Verification items for the finished model (mm, model axes). A direction names the side the tool comes from. Give positions to 0.01 mm unless a question says otherwise; leave off trailing zeros. Loops run counter-clockwise (first coordinate to the right, second up) from the corner with the lowest first, then second, coordinate; pieces in that order, holes last. Notation, with made-up numbers: M -29,54.5 L -24,54.5 A23 ccw -24,90.5 Z; hole C 72.5,13.25 d9. An arc over 180 degrees is marked long. Answer in a Markdown table with one row per item.
```python
from build123d import *

# Parameters (mm, degrees)
BOSS_EXTRUDE1_DEPTH      = 40
BOSS_EXTRUDE1_DEPTH_BACK = 40
CUT_EXTRUDE1_DEPTH       = 30
CUT_EXTRUDE1_DEPTH_BACK  = 48.5
SKETCH3_R                = 1.5
CUT_EXTRUDE2_DEPTH       = 40.921431767
FILLET1_R                = 1
CUT_EXTRUDE3_DEPTH       = 40
FILLET2_R                = 0.5


with BuildPart() as part:
    # Sketch1 → Boss-Extrude1 (new body, two sides)
    with BuildSketch(Plane(origin=(61.148873397, 0, -61.148873397), x_dir=(0.707106781, 0, 0.707106781), z_dir=(-0.707106781, 0, 0.707106781))) as boss_extrude1_sk:
        Polygon((-3.75, -92.901515315), (-3.75, -84.066578824), (-7.75, -81.757177748), (-7.75, -79.151515315), (3.75, -79.151515315), (3.75, -92.901515315), (3.75, -159.151515315), (-3.75, -159.151515315), align=None)
    extrude(amount=BOSS_EXTRUDE1_DEPTH)
    extrude(boss_extrude1_sk.sketch, amount=-BOSS_EXTRUDE1_DEPTH_BACK)

    # Sketch2 → Cut-Extrude1 (cut, two sides)
    with BuildSketch(Plane(origin=(-2.651650429, 0, -2.651650429), x_dir=(-0.707106781, 0, 0.707106781), z_dir=(-0.707106781, 0, -0.707106781))) as cut_extrude1_sk:
        with BuildLine():
            Line((-83.584702548, -79.151515315), (-83.584702548, -93.901515315))
            ThreePointArc((-83.584702548, -93.901515315), (-95.268174411, -132.944313121), (-126.477566081, -159.151515315))
            Line((-126.477566081, -159.151515315), (-126.477566081, -79.151515315))
            Line((-126.477566081, -79.151515315), (-83.584702548, -79.151515315))
        make_face()
        with BuildLine():
            Line((-65.634702548, -93.901515315), (-65.634702548, -79.151515315))
            Line((-65.634702548, -79.151515315), (-46.477566081, -79.151515315))
            Line((-46.477566081, -79.151515315), (-46.477566081, -159.151515315))
            Line((-46.477566081, -159.151515315), (-103.655823441, -159.151515315))
            ThreePointArc((-103.655823441, -159.151515315), (-75.833406523, -131.661176774), (-65.634702548, -93.901515315))
        make_face()
    extrude(amount=CUT_EXTRUDE1_DEPTH, mode=Mode.SUBTRACT)
    extrude(cut_extrude1_sk.sketch, amount=-CUT_EXTRUDE1_DEPTH_BACK, mode=Mode.SUBTRACT)

    # Sketch3 → Cut-Extrude2 (cut, through all)
    with BuildSketch(Plane(origin=(2.651650429, 0, 2.651650429), x_dir=(0.707106781, 0, -0.707106781), z_dir=(0.707106781, 0, 0.707106781))):
        with Locations((74.128214207, -88.901515315)):
            Circle(SKETCH3_R)
    extrude(amount=-CUT_EXTRUDE2_DEPTH, mode=Mode.SUBTRACT)

    # Fillet1
    fillet1_edges = [part.edges().sort_by_distance(p)[0] for p in [
        (73.295735665, -159.151515315, -73.295735665),
        (89.433144644, -159.151515315, -89.433144644),
    ]]
    fillet(fillet1_edges, radius=FILLET1_R)

    # Sketch4 → Cut-Extrude3 (cut)
    with BuildSketch(Plane(origin=(-2.651650429, 0, -2.651650429), x_dir=(-0.707106781, 0, 0.707106781), z_dir=(-0.707106781, 0, -0.707106781))):
        with BuildLine():
            ThreePointArc((-96.334442354, -150.659659636), (-100.301370683, -153.543969496), (-104.455461262, -156.151515315))
            Line((-104.455461262, -156.151515315), (-114.508069897, -156.151515315))
            ThreePointArc((-114.508069897, -156.151515315), (-107.203125114, -150.779152155), (-100.609312238, -144.554512732))
            Line((-100.609312238, -144.554512732), (-96.334442354, -150.659659636))
        make_face()
        with BuildLine():
            ThreePointArc((-85.691714117, -140.433955852), (-89.676742116, -144.76688928), (-94.002421329, -148.759790428))
            Line((-94.002421329, -148.759790428), (-98.550711636, -142.264158692))
            ThreePointArc((-98.550711636, -142.264158692), (-98.225553246, -141.884323374), (-97.902966063, -141.502301965))
            Line((-97.902966063, -141.502301965), (-85.691714117, -140.433955852))
        make_face()
        with BuildLine():
            ThreePointArc((-83.105887337, -137.19626581), (-82.806616537, -136.795716185), (-82.510134547, -136.393097949))
            Line((-82.510134547, -136.393097949), (-90.024605255, -130.087708349))
            ThreePointArc((-90.024605255, -130.087708349), (-92.547245897, -134.264707863), (-95.339415884, -138.266560873))
            Line((-95.339415884, -138.266560873), (-83.105887337, -137.19626581))
        make_face()
        with BuildLine():
            ThreePointArc((-80.784042437, -133.925239334), (-77.121371127, -127.814001685), (-74.080630429, -121.370688662))
            Line((-74.080630429, -121.370688662), (-88.136449193, -126.48658831))
            ThreePointArc((-88.136449193, -126.48658831), (-88.357906284, -126.934873492), (-88.582384151, -127.381653678))
            Line((-88.582384151, -127.381653678), (-80.784042437, -133.925239334))
        make_face()
        with BuildLine():
            Line((-82.791324081, -111.847238704), (-72.34560503, -116.718157493))
            ThreePointArc((-72.34560503, -116.718157493), (-72.505700586, -117.19183716), (-72.669081723, -117.664393631))
            Line((-72.669081723, -117.664393631), (-86.395070265, -122.660244896))
            ThreePointArc((-86.395070265, -122.660244896), (-84.384922058, -117.323155489), (-82.791324081, -111.847238704))
        make_face()
        with BuildLine():
            ThreePointArc((-68.79275862, -98.669648347), (-69.713665767, -106.319507983), (-71.446777789, -113.827153762))
            Line((-71.446777789, -113.827153762), (-82.109684478, -108.854958715))
            ThreePointArc((-82.109684478, -108.854958715), (-82.008492364, -108.355301003), (-81.910741312, -107.854958715))
            Line((-81.910741312, -107.854958715), (-68.79275862, -98.669648347))
        make_face()
        with BuildLine():
            ThreePointArc((-68.634702548, -93.901515315), (-68.636438764, -94.401527372), (-68.641647327, -94.901515315))
            Line((-68.641647327, -94.901515315), (-81.238542868, -103.721956531))
            ThreePointArc((-81.238542868, -103.721956531), (-80.748343571, -98.82260697), (-80.584702548, -93.901515315))
            Line((-80.584702548, -93.901515315), (-68.634702548, -93.901515315))
        make_face()
    extrude(amount=-CUT_EXTRUDE3_DEPTH, mode=Mode.SUBTRACT)

    # Fillet2
    fillet2_edges = [part.edges().sort_by_distance(p)[0] for p in [
        (68.11873745, -150.659659636, -68.11873745),
        (73.86116499, -156.151515315, -73.86116499),
        (80.969432725, -156.151515315, -80.969432725),
        (71.141526934, -144.554512732, -71.141526934),
        (60.593192144, -140.433955852, -60.593192144),
        (66.46974957, -148.759790428, -66.46974957),
        (69.685876488, -142.264158692, -69.685876488),
        (69.227851202, -141.502301965, -69.227851202),
        (58.343475655, -136.393097949, -58.343475655),
        (58.764736493, -137.19626581, -58.764736493),
        (67.415147486, -138.266560873, -67.415147486),
        (63.65700885, -130.087708349, -63.65700885),
        (52.382916131, -121.370688662, -52.382916131),
        (57.122944219, -133.925239334, -57.122944219),
        (62.637204527, -127.381653678, -62.637204527),
        (62.321880894, -126.48658831, -62.321880894),
        (58.542306681, -111.847238704, -58.542306681),
        (51.156067906, -116.718157493, -51.156067906),
        (51.384800469, -117.664393631, -51.384800469),
        (61.090540045, -122.660244896, -61.090540045),
        (48.643826116, -98.669648347, -48.643826116),
        (50.520501068, -113.827153762, -50.520501068),
        (58.060314695, -108.854958715, -58.060314695),
        (57.919640634, -107.854958715, -57.919640634),
        (48.532063596, -93.901515315, -48.532063596),
        (48.536974297, -94.901515315, -48.536974297),
        (57.444324556, -103.721956531, -57.444324556),
        (56.981989631, -93.901515315, -56.981989631),
    ]]
    fillet(fillet2_edges, radius=FILLET2_R)


solid = part.part
```
Item 1: Tool access check on faces 4 (the flat face through (54.931, -121.434, -60.235)), 5 (the flat face through (69.58, -147.63, -69.66)), 6 (the flat face through (47.19, -80.47, -58.15)). Record the directions out of +Z, -Z, +X, -X, +Y, -Y that give a thin tool (end or side, any length) a straight path to the whole face; none if there is none.
Reported:
| item | result |
|---|---|
| face 4 | -Z, -X, -Y |
| face 5 | none |
| face 6 | -Z, -X, +Y, -Y |
Item 2: Sectioned sample at A-A (y = -124). Record the cut outline in (x, z).
Reported:
| item | result |
|---|---|
| outline | M 48.22,-53.52 L 50.54,-55.85 L 55.85,-50.54 L 53.52,-48.22 Z; M 54.84,-60.14 L 61.18,-66.48 L 66.48,-61.18 L 60.14,-54.84 Z |
Item 3: Go/stop test with flat-tipped pins: pin 1 (1 mm diameter, centred on x = 64.5, z = -63.5, fed in from -Y); pin 2 (5.5 mm diameter, centred on x = 76.5, z = -75, fed in from +Y); pin 3 (10.5 mm diameter, centred on x = 56, z = -52, fed in from -Y). Record where each tip stops, or that it passes through.
Reported:
| item | result |
|---|---|
| pin 1 | stops at y = -150.14 |
| pin 2 | stops at y = -144.13 |
| pin 3 | stops at y = -140.18 |
Item 4: Scan lines: L1, parallel to Y at x = 63, z = -61.5; L2, parallel to Z at x = 51, y = -101; L3, parallel to Z at x = 50, y = -128.5. Record each from-to range of solid material in increasing order. Write a range as [from, to].
Reported:
| item | result |
|---|---|
| L1 | y = [-147.36, -143.07], [-140.64, -137.63], [-131.76, -127.84], [-126.46, -118.66] |
| L2 | z = [-56.3, -50.99], [-46.56, -45.7] |
| L3 | z = [-55.3, -54.78] |
Item 5: Release check for a two-part mould opening along X. For faces 1 (the flat face through (45.96, -86.63, -46.86)), 2 (the flat face through (55.84, -119.98, -55.92)), 3 (the flat face through (58.65, -86.423, -59.557)) record: released by +X, released by -X, zero draft, split by the parting line, or undercut.
Reported:
| item | result |
|---|---|
| face 1 | released by -X |
| face 2 | undercut |
| face 3 | released by +X |
